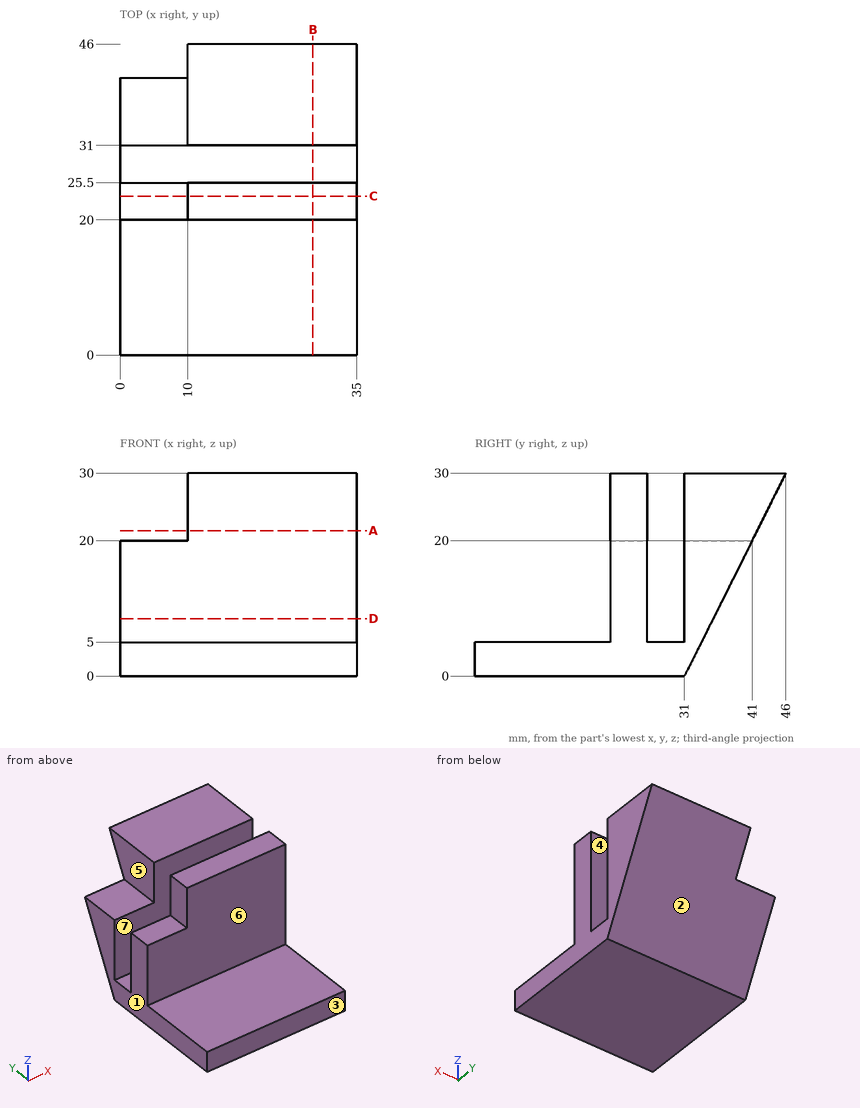
Job drawing, mm, ordinate dimensions from the low corner. One solid piece. A direction names the side the tool comes from. Round coordinates to 2 decimals unless told otherwise and drop trailing zeros. Write each loop counter-clockwise with the first axis right and the second up, starting at its lowest first coordinate (ties: lowest second). Pieces come first, ordered by that corner, then holes. Notation, with made-up numbers: M 19,-20 L 46,-20 A17 cw 46,9 Z; hole C 40.25,54.25 d3. An arc over 180 degrees is marked long. Return JSON: item names as keys, results as strings. Group by question number.
(1) Pin check, flat tips, straight feed: pin 1 Ø12.5 at (x, z) = (16.5, 15.5) entering from -Y; pin 2 Ø12 at (x, z) = (14.5, 12.5) entering from +Y; pin 3 Ø4.5 at (x, y) = (3, 24) entering from +Z; pin 4 Ø10 at (y, z) = (17, 21) entering from -X. Stop position of each tip, or through.
(2) Saw through at D-D on z = 8.5. Write the cut outline in (x, y).
(3) Which spindle directions (+Z, -Z, +X, -X, +Y, -Y) get a long thin tool onto all of the face, cutting with end or side? Do the marked faces 5, 6 and 7. Say none if no direction does.
(4) Saw through at A-A on z = 21.5. Write the cut outline in (x, y), then the cut area to 3 significant figures.
(5) Drill centre lines: probe 1 along Z at (x, y) = (3, 13); probe 2 along Y at (x, z) = (33, 25); probe 3 along Y at (x, z) = (2, 13). Where is each one in solid material? Low to high.
(6) Two-plate mould, pull along Y, no slides. Class the marked faces 1, 2, 3 and 4: +Y half, -Y half, draft (parallel to the pull), parting line (faces both ways), or undercut.
(7) Saw through at C-C on y = 23.5. Write the cut outline in (x, z).
(8) Saw through at B-B on x = 28.5. Write the cut outline in (y, z).
Returned:
{
 "1": {"pin 1": "y = 20", "pin 2": "y = 40.25", "pin 3": "z = 20", "pin 4": "x = 0"},
 "2": {"outline": "M 0,20 L 35,20 L 35,25.5 L 0,25.5 Z; M 0,31 L 35,31 L 35,35.25 L 0,35.25 Z"},
 "3": {"face 5": "+Z, -X, +Y, -Y", "face 6": "+Z, +X, -X, -Y", "face 7": "+Z, +X, -X"},
 "4": {"outline": "M 10,20 L 35,20 L 35,25.5 L 10,25.5 Z; M 10,31 L 35,31 L 35,41.75 L 10,41.75 Z", "area": "406 mm²"},
 "5": {"probe 1": "0 to 5", "probe 2": "20 to 25.5, 31 to 43.5", "probe 3": "20 to 25.5, 31 to 37.5"},
 "6": {"face 1": "draft", "face 2": "+Y half", "face 3": "-Y half", "face 4": "undercut"},
 "7": {"outline": "M 0,0 L 35,0 L 35,30 L 10,30 L 10,20 L 0,20 Z"},
 "8": {"outline": "M 0,0 L 31,0 L 46,30 L 31,30 L 31,5 L 25.5,5 L 25.5,30 L 20,30 L 20,5 L 0,5 Z"}
}
